Answer from the drawing. Dimensions are ordinates in mm from the lowest x, y and z of the part. A direction names the side the tool comes from. Round coordinates to 2 decimals unless told otherwise and drop trailing zeros. Loops run counter-clockwise (first coordinate to the right, second up) from the corner with the lowest first, then second, coordinate; pieces in that order, holes last. Notation, with made-up numbers: M -31,-8.5 L 8,-8.5 A26 ccw 8,11.5 Z; hole C -14.5,83 d10. An arc over 180 degrees is marked long. Answer as CSV lines item,"result".
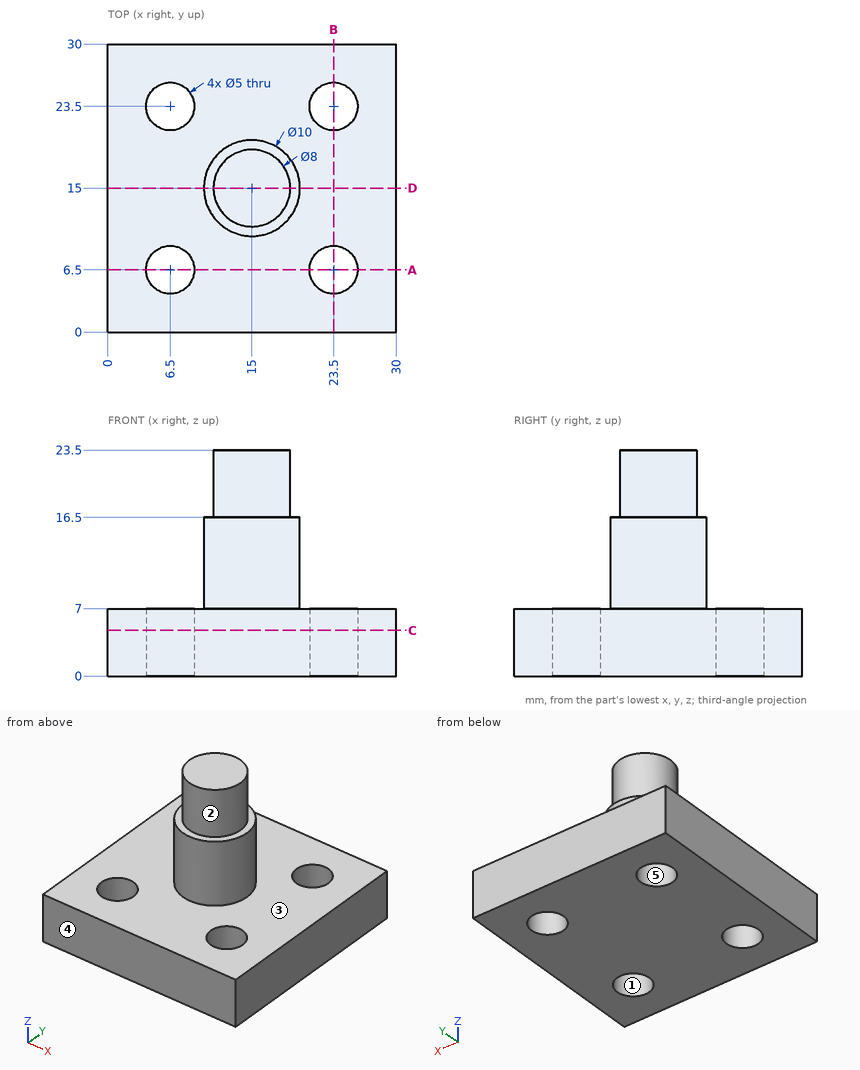
1) Find section D-D, the plane y = 15. Give the vertices of the cut face in (x, z), then the cut area to 3 significant figures.
Evaluation:
outline,"M 0,0 L 30,0 L 30,7 L 20,7 L 20,16.5 L 19,16.5 L 19,23.5 L 11,23.5 L 11,16.5 L 10,16.5 L 10,7 L 0,7 Z"
area,"361 mm^2"
2) A tool of negligible diameter and unlimited length cuts with its end or side. For the marked faces 1 and 2, from which of +Z, -Z, +X, -X, +Y, -Y can it reach the whole face along a straight path? Write none if from no direction.
Evaluation:
face 1,"+Z, -Z"
face 2,"+Z"
3) Each of these flat-tipped pins is pushed along its axis until it touches: P1, Ø4, axis at x = 23.5, y = 23.5, coming from the -Z side; P2, Ø2, axis at x = 16, z = 21, coming from the -Y side; P3, Ø4, axis at x = 10.5, y = 8, coming from the +Z side. Where does it stop, or does it pass through?
Evaluation:
P1,"passes through"
P2,"stops at y = 11"
P3,"stops at z = 7"
4) Determine the mould class of the marked faces 3, 4 and 5 for opening direction Y: released by +Y, released by -Y, zero draft, split by the parting line, or undercut.
Evaluation:
face 3,"zero draft"
face 4,"released by -Y"
face 5,"undercut"
5) Find section A-A, the plane y = 6.5. Give the vertices of the cut face in (x, z).
Evaluation:
outline,"M 0,0 L 4,0 L 4,7 L 0,7 Z; M 9,0 L 21,0 L 21,7 L 9,7 Z; M 26,0 L 30,0 L 30,7 L 26,7 Z"
6) Find section C-C, the plane z = 4.75. Give the vertices of the cut face in (x, y), then the cut area to 3 significant figures.
Evaluation:
outline,"M 0,0 L 30,0 L 30,30 L 0,30 Z; hole C 6.5,6.5 d5; hole C 6.5,23.5 d5; hole C 23.5,6.5 d5; hole C 23.5,23.5 d5"
area,"821 mm^2"
7) Straight lines are drawn through the part: line 1 (Y direction, x = 6.5, z = 3.75); line 2 (Y direction, x = 5.5, z = 4.5); line 3 (X direction, y = 8.5, z = 2.75). For each, find the intervals that lie inside material, in ascending order.
Evaluation:
line 1,"y = 0 to 4, 9 to 21, 26 to 30"
line 2,"y = 0 to 4.21, 8.79 to 21.21, 25.79 to 30"
line 3,"x = 0 to 5, 8 to 22, 25 to 30"
